Can you work these out from the model? Positions are in its coordinate system, mm. Coordinates: 2 decimals unless noted, no trailing zeros. Write each loop counter-clockwise with the first axis right and the second up, starting at its lowest first coordinate (ties: lowest second). Pieces come first, ordered by that corner, then holes. Notation, with made-up numbers: (17, -30.75) - (41, -30.75) arc R37 ccw to (41, 6.25) - close; hole circle Ø7 at (34.25, 45.25). An arc over 180 degrees is marked (long way). Use one line per item in the form item = value. Start each with the question number.
(1) If I drill on probe 1 along Z at (x, y) = (1.9, 60.96); probe 2 along Y at (x, z) = (1.55, 40.64); probe 3 along Z at (x, y) = (1, 20.32), over which ranges is the centre line in solid material (lowest first)? Write a range as from..to.
(2) For pin 1 Ø1.4 at (x, z) = (1.5, -0.5) entering from -Y, with a flat end and sliding along its axis, tell me the tip position at first contact or that it passes through.
(3) If we section it at C-C on y = 60.96: Please give me the cut outline in (x, z), then the cut area to 3 significant figures.
(4) If we section it at A-A on y = 20.32: Please give me the cut outline in (x, z), then the cut area to 3 significant figures.
(5) If we section it at B-B on z = -40.64: Please give me the cut outline in (x, y), then the cut area to 3 significant figures.
(6) If we section it at D-D on x = 1.4: Please give me the cut outline in (y, z) (3 decimals).
Autodesk Inventor part; units mm, degrees
ref_plane "YZ Plane" through (0, 0, 0) normal (1, 0, 0) x (0, 1, 0)
ref_plane "XZ Plane" through (0, 0, 0) normal (0, 1, 0) x (-1, 0, 0)
ref_plane "XY Plane" through (0, 0, 0) normal (0, 0, 1) x (1, 0, 0)
sketch "Sketch1" plane through (0, 0, 0) normal (1, 0, 0) x (0, 1, 0)
  line L0 (0, 45.72) -> (66.04, 45.72)
  line L1 (66.04, 45.72) -> (66.04, -45.72)
  line L2 (66.04, -45.72) -> (0, -45.72)
  line L3 (0, 35.56) -> (55.88, 35.56)
  line L4 (55.88, 35.56) -> (55.88, -35.56)
  line L5 (55.88, -35.56) -> (0, -35.56)
  line L6 (55.88, 35.56) -> (66.04, 45.72) construction
  line L7 (55.88, -35.56) -> (66.04, -45.72) construction
  line L8 (0, 45.72) -> (0, -45.72) construction
  line L9 (0, -45.72) -> (0, -35.56)
  line L10 (0, 35.56) -> (0, 45.72)
  point P0 (0, 0)
  point P1 (60.96, 40.64)
  point P2 (60.96, -40.64)
  point P3 (20.32, -40.64)
  point P4 (20.32, 40.64)
  point P5 (0, 0)
  dimension "d0" = 71.12
  dimension "d1" = 10.16
  dimension "d2" = 10.16
  dimension "d3" = 10.16
  dimension "d4" = 66.04
  dimension "d7" = 40.64
extrude "Extrusion2" add sketch "Sketch1" along normal blind 2.794
hole "Hole2" at (0, 60.96, 40.64) at (0, 60.96, -40.64) at (0, 20.32, -40.64) at (0, 20.32, 40.64) direction (1, 0, 0) diameter 4 end through all
fillet "Fillet1" radius 3.175 6 edges at (1.397, 0, -35.56) (1.397, 0, 35.56) (1.397, 0, -45.72) (1.397, 0, 45.72) (1.397, 66.04, 45.72) (1.397, 66.04, -45.72)
equation "\"d2\" = d1"
equation "\"d3\" = d2"
properties part number "ArmSpacer" material "Polycarbonate, Smoke"
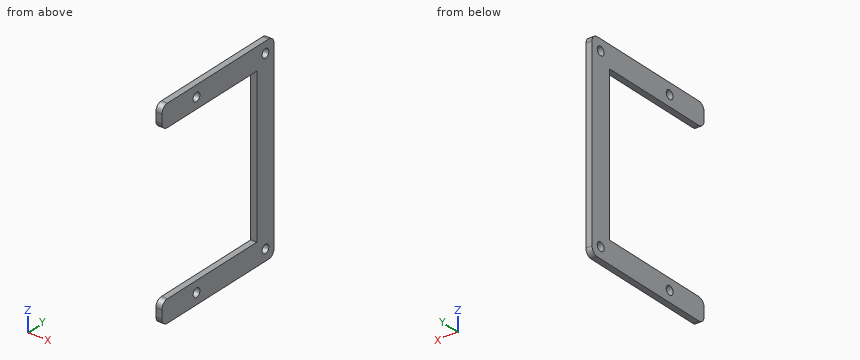
Reported:
q1.probe_1 = -45.72..-42.64, -38.64..38.64, 42.64..45.72
q1.probe_2 = 0..18.32, 22.32..58.96, 62.96..66.04
q1.probe_3 = -45.72..-42.64, -38.64..-35.56, 35.56..38.64, 42.64..45.72
q2.pin_1 = 55.88
q3.outline = (0, -45.72) - (2.79, -45.72) - (2.79, -42.64) - (0, -42.64) - close; (0, -38.64) - (2.79, -38.64) - (2.79, 38.64) - (0, 38.64) - close; (0, 42.64) - (2.79, 42.64) - (2.79, 45.72) - (0, 45.72) - close
q3.area = 233 mm2
q4.outline = (0, -45.72) - (2.79, -45.72) - (2.79, -42.64) - (0, -42.64) - close; (0, -38.64) - (2.79, -38.64) - (2.79, -35.56) - (0, -35.56) - close; (0, 35.56) - (2.79, 35.56) - (2.79, 38.64) - (0, 38.64) - close; (0, 42.64) - (2.79, 42.64) - (2.79, 45.72) - (0, 45.72) - close
q4.area = 34.4 mm2
q5.outline = (0, 0) - (2.79, 0) - (2.79, 18.32) - (0, 18.32) - close; (0, 22.32) - (2.79, 22.32) - (2.79, 58.96) - (0, 58.96) - close; (0, 62.96) - (2.79, 62.96) - (2.79, 66.04) - (0, 66.04) - close
q5.area = 162 mm2
q6.outline = (0, -42.545) arc R3.175 ccw to (3.175, -45.72) - (62.865, -45.72) arc R3.175 ccw to (66.04, -42.545) - (66.04, 42.545) arc R3.175 ccw to (62.865, 45.72) - (3.175, 45.72) arc R3.175 ccw to (0, 42.545) - (0, 38.735) arc R3.175 ccw to (3.175, 35.56) - (55.88, 35.56) - (55.88, -35.56) - (3.175, -35.56) arc R3.175 ccw to (0, -38.735) - close; hole circle Ø4 at (20.32, -40.64); hole circle Ø4 at (20.32, 40.64); hole circle Ø4 at (60.96, -40.64); hole circle Ø4 at (60.96, 40.64)
